```python
from build123d import *

# Parameters (mm, degrees)
SKETCH1_R           = 3.175
SKETCH1_R_2         = 1.27
BOSS_EXTRUDE1_DEPTH = 3.175
CUT_EXTRUDE1_DEPTH  = 3.175
FILLET1_R           = 6.35
SKETCH3_W           = 9.525
SKETCH3_H           = 9.525
BOSS_EXTRUDE2_DEPTH = 3.175
FILLET2_R           = 1.5875
SKETCH4_R           = 3.175
SKETCH4_R_2         = 1.27
BOSS_EXTRUDE3_DEPTH = 9.525
SKETCH5_W           = 3.175
SKETCH5_H           = 6.35
BOSS_EXTRUDE4_DEPTH = 9.525
FILLET4_R           = 2.54


with BuildPart() as part:
    # Sketch1 → Boss-Extrude1 (new body)
    with BuildSketch(Plane(origin=(0, 0, 0), x_dir=(1, 0, 0), z_dir=(0, 1, 0))):
        Polygon((-82.55, 31.75), (-82.55, -44.45), (44.45, -44.45), (44.45, 4.889379277), (-57.15, 31.75), align=None)
        Circle(SKETCH1_R, mode=Mode.SUBTRACT)
        with Locations((0, 12.7)):
            Circle(SKETCH1_R_2, mode=Mode.SUBTRACT)
        with Locations((12.7, 0)):
            Circle(SKETCH1_R_2, mode=Mode.SUBTRACT)
        with Locations((0, -12.7)):
            Circle(SKETCH1_R_2, mode=Mode.SUBTRACT)
        with Locations((-12.7, 0)):
            Circle(SKETCH1_R_2, mode=Mode.SUBTRACT)
        with Locations((-57.15, 25.774227063)):
            Circle(SKETCH1_R_2, mode=Mode.SUBTRACT)
        with Locations((-76.2, 25.4)):
            Circle(SKETCH1_R_2, mode=Mode.SUBTRACT)
        with Locations((38.1, 0)):
            Circle(SKETCH1_R_2, mode=Mode.SUBTRACT)
    extrude(amount=BOSS_EXTRUDE1_DEPTH)

    # Sketch2 → Cut-Extrude1 (cut)
    with BuildSketch(Plane(origin=(0, 3.175, 0), x_dir=(1, 0, 0), z_dir=(0, 1, 0))):
        with BuildLine():
            Line((-69.85, 10.16), (-69.85, -29.21))
            ThreePointArc((-69.85, -29.21), (-69.106051224, -31.006051224), (-67.31, -31.75))
            Line((-67.31, -31.75), (-12.065, -31.75))
            ThreePointArc((-12.065, -31.75), (-10.268948776, -31.006051224), (-9.525, -29.21))
            Line((-9.525, -29.21), (-9.525, -17.904297668))
            ThreePointArc((-9.525, -17.904297668), (-9.822578777, -16.711340394), (-10.645588235, -15.797909707))
            ThreePointArc((-10.645588235, -15.797909707), (-18.486020774, -4.6010364), (-16.808823529, 8.964705882))
            ThreePointArc((-16.808823529, 8.964705882), (-16.871967969, 11.466819219), (-19.05, 12.7))
            Line((-19.05, 12.7), (-67.31, 12.7))
            ThreePointArc((-67.31, 12.7), (-69.106051224, 11.956051224), (-69.85, 10.16))
        make_face()
        with BuildLine():
            Line((9.525, -17.904297668), (9.525, -29.21))
            ThreePointArc((9.525, -29.21), (10.268948776, -31.006051224), (12.065, -31.75))
            Line((12.065, -31.75), (29.21, -31.75))
            ThreePointArc((29.21, -31.75), (31.006051224, -31.006051224), (31.75, -29.21))
            Line((31.75, -29.21), (31.75, -6.845130987))
            ThreePointArc((31.75, -6.845130987), (31.222535045, -5.295517264), (29.859210479, -4.38949955))
            Line((29.859210479, -4.38949955), (21.722749497, -2.23841301))
            ThreePointArc((21.722749497, -2.23841301), (19.753320798, -2.524108077), (18.594299133, -4.141803924))
            ThreePointArc((18.594299133, -4.141803924), (15.73877231, -10.732825637), (10.645588235, -15.797909707))
            ThreePointArc((10.645588235, -15.797909707), (9.822578777, -16.711340394), (9.525, -17.904297668))
        make_face()
    extrude(amount=-CUT_EXTRUDE1_DEPTH, mode=Mode.SUBTRACT)

    # Fillet1
    fillet1_edges = [part.edges().sort_by_distance(p)[0] for p in [
        (-57.15, 1.5875, -31.75),
        (44.45, 1.5875, -4.889379277),
        (-82.55, 1.5875, -31.75),
    ]]
    fillet(fillet1_edges, radius=FILLET1_R)

    # Sketch3 → Boss-Extrude2 (add)
    with BuildSketch(Plane.XY.offset(44.45)):
        with Locations((-77.7875, 7.9375)):
            Rectangle(SKETCH3_W, SKETCH3_H)
        Polygon((-77.7875, 5.243423164), (-75.093423164, 7.9375), (-77.7875, 10.631576836), (-80.481576836, 7.9375), align=None, mode=Mode.SUBTRACT)
        with Locations((39.6875, 7.9375)):
            Rectangle(SKETCH3_W, SKETCH3_H)
        Polygon((39.6875, 5.243423164), (42.381576836, 7.9375), (39.6875, 10.631576836), (36.993423164, 7.9375), align=None, mode=Mode.SUBTRACT)
        with Locations((-19.05, 7.9375)):
            Rectangle(SKETCH3_W, SKETCH3_H)
        Polygon((-19.05, 5.243423164), (-16.355923164, 7.9375), (-19.05, 10.631576836), (-21.744076836, 7.9375), align=None, mode=Mode.SUBTRACT)
    extrude(amount=-BOSS_EXTRUDE2_DEPTH)

    # Fillet2
    fillet2_edges = [part.edges().sort_by_distance(p)[0] for p in [
        (-82.55, 12.7, 42.8625),
        (-73.025, 12.7, 42.8625),
        (-77.7875, 3.175, 41.275),
        (-73.025, 3.175, 42.8625),
        (44.45, 12.7, 42.8625),
        (39.6875, 3.175, 41.275),
        (34.925, 3.175, 42.8625),
        (34.925, 12.7, 42.8625),
        (-23.8125, 3.175, 42.8625),
        (-23.8125, 12.7, 42.8625),
        (-14.2875, 12.7, 42.8625),
        (-19.05, 3.175, 41.275),
        (-14.2875, 3.175, 42.8625),
    ]]
    fillet(fillet2_edges, radius=FILLET2_R)

    # Sketch4 → Boss-Extrude3 (add)
    with BuildSketch(Plane(origin=(0, 3.175, 0), x_dir=(1, 0, 0), z_dir=(0, 1, 0))):
        with Locations((-76.2, 25.4)):
            Circle(SKETCH4_R)
        with Locations((-76.2, 25.4)):
            Circle(SKETCH4_R_2, mode=Mode.SUBTRACT)
        with Locations((38.1, 0)):
            Circle(SKETCH4_R)
        with Locations((38.1, 0)):
            Circle(SKETCH4_R_2, mode=Mode.SUBTRACT)
    extrude(amount=BOSS_EXTRUDE3_DEPTH)

    # Sketch5 → Boss-Extrude4 (add)
    with BuildSketch(Plane(origin=(0, 3.175, 0), x_dir=(1, 0, 0), z_dir=(0, 1, 0))):
        with Locations((8.751486047, -36.616058846)):
            Rectangle(SKETCH5_W, SKETCH5_H)
    extrude(amount=BOSS_EXTRUDE4_DEPTH)

    # Fillet4
    fillet4_edges = [part.edges().sort_by_distance(p)[0] for p in [
        (-79.375, 3.175, -25.4),
        (34.925, 3.175, 0),
    ]]
    fillet(fillet4_edges, radius=FILLET4_R)


solid = part.part
```
Check sheet for the modelled part. Datum: model origin and axes. Units: mm. A direction names the side the tool comes from. Coordinates: 2 decimals unless noted, no trailing zeros. Write each loop counter-clockwise with the first axis right and the second up, starting at its lowest first coordinate (ties: lowest second). Pieces come first, ordered by that corner, then holes. Notation, with made-up numbers: M -9,85 L 40,85 A21 ccw 40,106 Z; hole C 0.5,68.5 d5. An arc over 180 degrees is marked long. Write item = value, one per line. Start each with the question number.
1. Thickness scan on probe 1 along X at (y, z) = (1.3, 0) (3 decimals); probe 2 along Z at (x, y) = (12.7, 2); probe 3 along Z at (x, y) = (-12.7, 0.7). Record the ranges inside material, lowest first.
2. Sectioned sample at A-A (z = 12.7). Record the cut outline in (x, y) (3 decimals), then the cut area to 3 significant figures.
3. Sectioned sample at C-C (x = 0). Record the cut outline in (y, z) (3 decimals), then the cut area to 3 significant figures.
4. Sectioned sample at D-D (y = 1.25). State how many separate pieces and enclosed holes the cut face has, then the cut area to 3 significant figures.
5. Tool access check on faces 1 (the flat face through (-17.722, 6.572, 42.885)), 2 (the flat face through (9, 8, 33.441)), 3 (the flat face through (-79.12, 9.3, 42.88)). Record the directions out of +Z, -Z, +X, -X, +Y, -Y that give a thin tool (end or side, any length) a straight path to the whole face; none if there is none.
6. Sectioned sample at B-B (x = -31.5). Record the cut outline in (y, z) (3 decimals).
7. Go/stop test with flat-tipped pins: pin 1 (1 mm diameter, centred on x = 8, y = 5.5, fed in from -Z); pin 2 (2.5 mm diameter, centred on x = -40.5, y = 2, fed in from -Z); pin 3 (3.5 mm diameter, centred on x = -12.7, z = 0, fed in from +Y) (3 decimals). Record where each tip stops, or that it passes through.
8. Mould release check, pull along Y, two halves, no side actions. Record for faces 4 (the flat face through (40, 12.7, 43)), 5 (the cylindrical face through (31.237, 1.61, 5.314)), 6 (the flat face through (-20.416, 6.609, 42.885)): pulls with the +Y half, pulls with the -Y half, needs draft (parallel to the pull), parting line crosses it, or undercut.
The answers:
q1.probe_1 = -82.55 to -69.85, -19.05 to -13.97, -11.43 to -3.175, 3.175 to 11.43, 13.97 to 36.83, 39.37 to 44.45
q1.probe_2 = -13.28 to -1.27, 1.27 to 14.2, 31.75 to 44.45
q1.probe_3 = -20 to -1.27, 1.27 to 14.2, 31.75 to 44.45
q2.outline = M -82.55,0 L -69.85,0 L -69.85,3.175 L -82.55,3.175 Z; M -14.199,0 L -1.27,0 L -1.27,3.175 L -14.199,3.175 Z; M 1.27,0 L 14.199,0 L 14.199,3.175 L 1.27,3.175 Z; M 31.75,0 L 44.45,0 L 44.45,3.175 L 31.75,3.175 Z
q2.area = 163 mm²
q3.outline = M 0,-16.641 L 3.175,-16.641 L 3.175,-13.97 L 0,-13.97 Z; M 0,-11.43 L 3.175,-11.43 L 3.175,-3.175 L 0,-3.175 Z; M 0,3.175 L 3.175,3.175 L 3.175,11.43 L 0,11.43 Z; M 0,13.97 L 3.175,13.97 L 3.175,44.45 L 0,44.45 Z
q3.area = 158 mm²
q4.separate_pieces = 1
q4.enclosed_holes = 10
q4.area = 5,230 mm²
q5.face_1 = +Z, -Z
q5.face_2 = -Z, +X, -X, +Y
q5.face_3 = +Z
q6.outline = M 0,-24.969 L 3.175,-24.969 L 3.175,-12.7 L 0,-12.7 Z; M 0,31.75 L 3.175,31.75 L 3.175,44.45 L 0,44.45 Z
q7.pin_1 = 33.44
q7.pin_2 = -27.68
q7.pin_3 = 3.175
q8.face_4 = pulls with the +Y half
q8.face_5 = needs draft
q8.face_6 = undercut
